```python
from build123d import *

# Parameters (mm, degrees)
BOSS_EXTRUDE1_DEPTH      = 23.01875
BOSS_EXTRUDE1_DEPTH_BACK = 16.66875
SKETCH8_OUTSIDE_W        = 7085.338
SKETCH8_OUTSIDE_H        = 7090.25
SKETCH8_OUTSIDE_R        = 15.875
CUT_EXTRUDE7_DEPTH       = 2032
CUT_EXTRUDE7_TAPER       = 60
SKETCH20_OUTSIDE_W       = 55.082
SKETCH20_OUTSIDE_H       = 59.994
SKETCH20_OUTSIDE_R       = 15.875
CUT_EXTRUDE9_DEPTH       = 2.54
CUT_EXTRUDE9_TAPER       = 60
CHAMFER1_SIZE2           = 1.101615862
CHAMFER1_SIZE            = 1.0668


with BuildPart() as part:
    # Sketch2 → Boss-Extrude1 (new body, two sides)
    with BuildSketch(Plane.XY) as boss_extrude1_sk:
        Polygon((0, 18.330871047), (-15.875, 9.165435523), (-15.875, -9.165435523), (0, -18.330871047), (15.875, -9.165435523), (15.875, 9.165435523), align=None)
    extrude(amount=BOSS_EXTRUDE1_DEPTH)
    extrude(boss_extrude1_sk.sketch, amount=-BOSS_EXTRUDE1_DEPTH_BACK)

    # Sketch5 → Cut-Revolve1 (revolve, cut)
    with BuildSketch(Plane(origin=(0, 0, 0), x_dir=(0, 0, -1), z_dir=(1, 0, 0))):
        Polygon((-23.01875, 0), (-23.01875, 14.2875), (0, 14.2875), (1.918229167, 11.43), (3.836458333, 11.43), (5.580126, 12.989754658), (16.66875, 13.335), (16.66875, 0), align=None)
    revolve(axis=Axis((0, 0, -16.66875), (0, 0, 1)), mode=Mode.SUBTRACT)

    # Sketch24 → Cut-Revolve2 (revolve, cut)
    with BuildSketch(Plane(origin=(0, 0, 0), x_dir=(0, 0, -1), z_dir=(1, 0, 0))):
        with BuildLine():
            Line((-23.01875, 15.5956), (-23.01875, 18.330871047))
            Line((-23.01875, 18.330871047), (3.439583333, 18.330871047))
            Line((3.439583333, 18.330871047), (3.439583333, 15.875))
            Line((3.439583333, 15.875), (-0.970138889, 15.875))
            ThreePointArc((-0.970138889, 15.875), (-4.278435497, 15.834225325), (-7.584722222, 15.71192607))
            ThreePointArc((-7.584722222, 15.71192607), (-9.943206753, 15.624685935), (-12.303125, 15.5956))
            Line((-12.303125, 15.5956), (-23.01875, 15.5956))
        make_face()
    revolve(axis=Axis((0, 0, 0), (0, 0, 1)), mode=Mode.SUBTRACT)

    # Sketch8 outside → Cut-Extrude7 (cut)
    with BuildSketch(Plane.XY.offset(-16.66875)):
        Rectangle(SKETCH8_OUTSIDE_W, SKETCH8_OUTSIDE_H)
        Circle(SKETCH8_OUTSIDE_R, mode=Mode.SUBTRACT)
    extrude(amount=CUT_EXTRUDE7_DEPTH, taper=CUT_EXTRUDE7_TAPER, mode=Mode.SUBTRACT)

    # Sketch20 outside → Cut-Extrude9 (cut)
    with BuildSketch(Plane(origin=(0, 0, -3.439583333), x_dir=(-1, 0, 0), z_dir=(0, 0, -1))):
        Rectangle(SKETCH20_OUTSIDE_W, SKETCH20_OUTSIDE_H)
        Circle(SKETCH20_OUTSIDE_R, mode=Mode.SUBTRACT)
    extrude(amount=CUT_EXTRUDE9_DEPTH, taper=CUT_EXTRUDE9_TAPER, mode=Mode.SUBTRACT)

    # Chamfer1
    chamfer1_edges = [part.edges().sort_by_distance(p)[0] for p in [
        (0, -13.335, -16.66875),
    ]]
    chamfer(chamfer1_edges, length=CHAMFER1_SIZE, length2=CHAMFER1_SIZE2)


solid = part.part
```
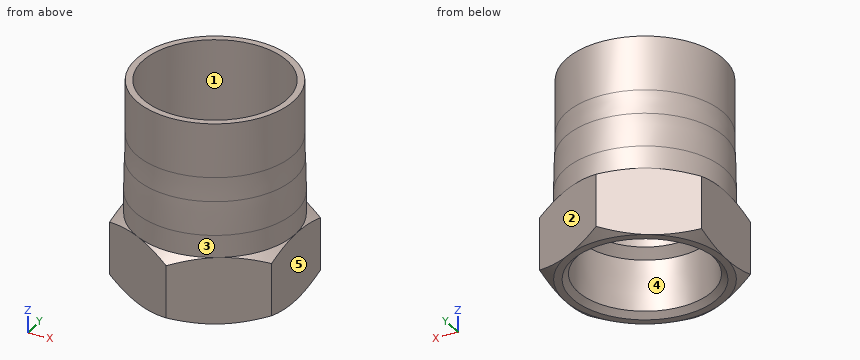
Source: CAD feature listing. Evaluate the final solid. Frame: model axes, mm. Face numbers are marked on the shaded views. A direction names the side the tool comes from. Coordinates: 2 decimals unless noted, no trailing zeros. Write each loop counter-clockwise with the first axis right and the second up, starting at its lowest first coordinate (ties: lowest second). Pieces come first, ordered by that corner, then holes. Notation, with made-up numbers: (-12.5, 40) -> (25.5, 40) arc R16 ccw to (25.5, 47) -> close; hole circle Ø9 at (17.5, -11). An arc over 180 degrees is marked (long way). Return JSON: item names as keys, results as strings. Group by question number.
1) Section query A-A, the plane z = -10. Return loops of the section in (x, y) (3 decimals), plus the area to 3 significant figures.
2) Mould query, pull axis X, two halves, no side actions, for the marked faces 3, 4 and 5. Classes: +X half, -X half, draft (parallel to the pull), parting line (faces both ways), or undercut.
3) Ray query, line 1 along Y through (x, z) = (0, 13); line 2 along X through (y, z) = (0, -3.15) (3 decimals). Return the intervals inside material, ascending.
4) Set-up query: the marked faces 1 and 2. Return all of +Z, -Z, +X, -X, +Y, -Y with unobstructed straight access to the full face (end or side cutting, diameter ignored); none if empty.
5) Contact query for flat-ended pins moving along their axis: P1, Ø12, axis at x = -3.5, y = -0.5, coming from the -Z side; P2, Ø12, axis at x = 6.5, z = -9.5, coming from the -Y side; P3, Ø8, axis at x = 1, z = 1, coming from the -Y side (3 decimals); P4, Ø1, axis at x = -9.5, z = -1, coming from the -Y side. Output: stop coordinate, or through.
From the geometry:
{
 "1": {"outline": "(-15.875, -9.165) -> (0, -18.331) -> (15.875, -9.165) -> (15.875, 9.165) -> (0, 18.331) -> (-15.875, 9.165) -> close; hole circle Ø26.255 at (0, 0)", "area": "332 mm²"},
 "2": {"face 3": "parting line", "face 4": "undercut", "face 5": "+X half"},
 "3": {"line 1": "-15.6 to -14.29, 14.29 to 15.6", "line 2": "-15.875 to -11.43, 11.43 to 15.875"},
 "4": {"face 1": "+Z", "face 2": "+Z, -Z, +X, +Y"},
 "5": {"P1": "through", "P2": "y = -18.04", "P3": "y = -15.875", "P4": "y = -13.08"}
}
